from build123d import *
from build123d.topology import SkipClean

# Parameters (mm, degrees)
EXTRUDE_1_DEPTH          = 20
EXTRUDE_2_DEPTH          = 35
FILLET_1_R               = 2
FILLET_2_R               = 2
SKETCH_3_W               = 55
SKETCH_3_H               = 8
EXTRUDE_3_DEPTH          = 20
CUT_EXTRUDE_1_DEPTH      = 81.785122448
FILLET_3_R               = 2
CUT_EXTRUDE_2_DEPTH      = 92.549767886
CUT_EXTRUDE_2_DEPTH_BACK = 92.549767886
SKETCH_6_R               = 3.05
CUT_EXTRUDE_3_DEPTH      = 5.1
FILLET_3_OF_MIRROR_1_R   = 2
CUT_EXTRUDE_4_DEPTH      = 75.837223358
CUT_EXTRUDE_4_DEPTH_BACK = 75.837223358
SKETCH_9_R               = 1.6
SKETCH_10_R              = 3
CUT_EXTRUDE_5_DEPTH      = 3
CUT_EXTRUDE_START        = -2
SKETCH_11_R              = 3
CUT_EXTRUDE_6_DEPTH      = 2
CUT_EXTRUDE_7_DEPTH      = 75.837223358
CUT_EXTRUDE_7_DEPTH_BACK = 75.837223358
SKETCH_12_W              = 29.59816484
SKETCH_12_H              = 37.248372047
SKETCH_12_W_2            = 30.6542071
SKETCH_12_H_2            = 41.472541085
SKETCH_13_W              = 45
SKETCH_13_H              = 8
EXTRUDE_4_DEPTH          = 20
CUT_EXTRUDE_8_DEPTH      = 69.398976601
CUT_EXTRUDE_8_DEPTH_BACK = 69.398976601
SKETCH_14_R              = 2.1
FILLET_5_R               = 1
FILLET_6_R               = 2


with BuildPart() as part:
    # 草图1 → 凸台-拉伸1 (new body)
    with BuildSketch(Plane.XY):
        with BuildLine():
            Line((-24.5, -24.4), (24.5, -24.4))
            Line((24.5, -24.4), (24.5, 15.6))
            ThreePointArc((24.5, 15.6), (0, 23.936691271), (-24.5, 15.6))
            Line((-24.5, 15.6), (-24.5, -24.4))
        make_face()
        with BuildLine():
            Line((-6.480740698, 9.5), (6.480740698, 9.5))
            ThreePointArc((6.480740698, 9.5), (8.131727984, 8.131727984), (9.5, 6.480740698))
            Line((9.5, 6.480740698), (9.5, -6.480740698))
            ThreePointArc((9.5, -6.480740698), (8.131727984, -8.131727984), (6.480740698, -9.5))
            Line((6.480740698, -9.5), (-6.480740698, -9.5))
            ThreePointArc((-6.480740698, -9.5), (-8.131727984, -8.131727984), (-9.5, -6.480740698))
            Line((-9.5, -6.480740698), (-9.5, 6.480740698))
            ThreePointArc((-9.5, 6.480740698), (-8.131727984, 8.131727984), (-6.480740698, 9.5))
        make_face(mode=Mode.SUBTRACT)
    extrude(amount=EXTRUDE_1_DEPTH)

    # 草图2 → 凸台-拉伸2 (add)
    with SkipClean():  # the faces are left unmerged after this step: merging them gives an invalid solid
        with BuildSketch(Plane.XY.offset(20)):
            with BuildLine():
                Line((-20.5, 18.311818868), (-20.5, -20.4))
                Line((-20.5, -20.4), (20.5, -20.4))
                Line((20.5, -20.4), (20.5, 18.311818868))
                ThreePointArc((20.5, 18.311818868), (22.540818317, 17.016117462), (24.5, 15.6))
                Line((24.5, 15.6), (24.5, -24.4))
                Line((24.5, -24.4), (-24.5, -24.4))
                Line((-24.5, -24.4), (-24.5, 15.6))
                ThreePointArc((-24.5, 15.6), (-22.540818317, 17.016117462), (-20.5, 18.311818868))
            make_face()
        extrude(amount=EXTRUDE_2_DEPTH)

    # 圆角1
    fillet_1_edges = [part.edges().sort_by_distance(p)[0] for p in [
        (-24.5, 15.6, 37.5),
        (24.5, 15.6, 37.5),
        (24.5, -24.4, 37.5),
        (-24.5, -24.4, 37.5),
    ]]
    fillet(fillet_1_edges, radius=FILLET_1_R)

    # 圆角2
    fillet_2_edges = [part.edges().sort_by_distance(p)[0] for p in [
        (8.131727984, 8.131727984, 20),
        (0, 9.5, 20),
        (-8.131727984, 8.131727984, 20),
        (-9.5, 0, 20),
        (-8.131727984, -8.131727984, 20),
        (0, -9.5, 20),
        (8.131727984, -8.131727984, 20),
        (9.5, 0, 20),
    ]]
    fillet(fillet_2_edges, radius=FILLET_2_R)

    # 草图3 → 凸台-拉伸3 (add)
    with SkipClean():  # the faces are left unmerged after this step: merging them gives an invalid solid
        with BuildSketch(Plane.ZY.offset(24.5)):
            with Locations((27.5, 10.599820628)):
                Rectangle(SKETCH_3_W, SKETCH_3_H)
            with Locations((27.5, -18.000179372)):
                Rectangle(SKETCH_3_W, SKETCH_3_H)
        extrude_3 = extrude(amount=EXTRUDE_3_DEPTH)

    # 草图4 → 切除-拉伸1 (cut, symmetric)
    with SkipClean():  # the faces are left unmerged after this step: merging them gives an invalid solid
        with BuildSketch(Plane(origin=(0, 14.599820628, 0), x_dir=(1, 0, 0), z_dir=(0, 1, 0))):
            with BuildLine():
                Line((-39.25, -11.75), (-29.75, -11.75))
                ThreePointArc((-29.75, -11.75), (-29.042893219, -12.042893219), (-28.75, -12.75))
                Line((-28.75, -12.75), (-28.75, -17.25))
                ThreePointArc((-28.75, -17.25), (-29.042893219, -17.957106781), (-29.75, -18.25))
                Line((-29.75, -18.25), (-39.25, -18.25))
                ThreePointArc((-39.25, -18.25), (-39.957106781, -17.957106781), (-40.25, -17.25))
                Line((-40.25, -17.25), (-40.25, -12.75))
                ThreePointArc((-40.25, -12.75), (-39.957106781, -12.042893219), (-39.25, -11.75))
            make_face()
            with BuildLine():
                Line((-39.25, -36.75), (-29.75, -36.75))
                ThreePointArc((-29.75, -36.75), (-29.042893219, -37.042893219), (-28.75, -37.75))
                Line((-28.75, -37.75), (-28.75, -42.25))
                ThreePointArc((-28.75, -42.25), (-29.042893219, -42.957106781), (-29.75, -43.25))
                Line((-29.75, -43.25), (-39.25, -43.25))
                ThreePointArc((-39.25, -43.25), (-39.957106781, -42.957106781), (-40.25, -42.25))
                Line((-40.25, -42.25), (-40.25, -37.75))
                ThreePointArc((-40.25, -37.75), (-39.957106781, -37.042893219), (-39.25, -36.75))
            make_face()
        cut_extrude_1 = extrude(amount=CUT_EXTRUDE_1_DEPTH, both=True, mode=Mode.SUBTRACT)

    # 圆角3
    fillet_3_edges = [part.edges().sort_by_distance(p)[0] for p in [
        (-44.5, 6.599820628, 27.5),
        (-44.5, 14.599820628, 27.5),
        (-44.5, -14.000179372, 27.5),
        (-44.5, -22.000179372, 27.5),
    ]]
    fillet(fillet_3_edges, radius=FILLET_3_R)

    # 草图6 → 切除-拉伸2 (cut, two sides: drawn at the far end of the back side and taken through both)
    with BuildSketch(Plane(origin=(24.5, 0, 0), x_dir=(0, 0, -1), z_dir=(1, 0, 0)).offset(-CUT_EXTRUDE_2_DEPTH_BACK)):
        with Locations(Location((-10.4, 0, 0), (0, 0, 270))):
            Circle(SKETCH_6_R)
    extrude(amount=CUT_EXTRUDE_2_DEPTH + CUT_EXTRUDE_2_DEPTH_BACK, mode=Mode.SUBTRACT)

    # 草图7 → 切除-拉伸3 (cut)
    with BuildSketch(Plane(origin=(24.5, 0, 0), x_dir=(0, 0, -1), z_dir=(1, 0, 0))):
        Polygon((-5.4, -2.886751346), (-5.4, 2.886751346), (-10.4, 5.773502692), (-15.4, 2.886751346), (-15.4, -2.886751346), (-10.4, -5.773502692), align=None)
    cut_extrude_3 = extrude(amount=-CUT_EXTRUDE_3_DEPTH, mode=Mode.SUBTRACT)

    # 镜向1: 凸台-拉伸3, 切除-拉伸1, 切除-拉伸3 across plane
    add(extrude_3.mirror(Plane(origin=(0, 0, 0), x_dir=(0, 0, 1), z_dir=(1, 0, 0))))
    add(cut_extrude_1.mirror(Plane(origin=(0, 0, 0), x_dir=(0, 0, 1), z_dir=(1, 0, 0))), mode=Mode.SUBTRACT)
    add(cut_extrude_3.mirror(Plane(origin=(0, 0, 0), x_dir=(0, 0, 1), z_dir=(1, 0, 0))), mode=Mode.SUBTRACT)

    # 圆角3 of 镜向1
    fillet_3_of_mirror_1_edges = [part.edges().sort_by_distance(p)[0] for p in [
        (44.5, 6.599820628, 27.5),
        (44.5, 14.599820628, 27.5),
        (44.5, -14.000179372, 27.5),
        (44.5, -22.000179372, 27.5),
    ]]
    fillet(fillet_3_of_mirror_1_edges, radius=FILLET_3_OF_MIRROR_1_R)

    # 草图9 → 切除-拉伸4 (cut, two sides: drawn at the far end of the back side and taken through both)
    with BuildSketch(Plane(origin=(0, 0, 0), x_dir=(-1, 0, 0), z_dir=(0, 0, -1)).offset(-CUT_EXTRUDE_4_DEPTH_BACK)):
        with Locations((34.5, -18.000179372)):
            Circle(SKETCH_9_R)
        with Locations((34.5, 10.599820628)):
            Circle(SKETCH_9_R)
        with Locations((-34.5, 10.599820628)):
            Circle(SKETCH_9_R)
        with Locations((-34.5, -18.000179372)):
            Circle(SKETCH_9_R)
    extrude(amount=CUT_EXTRUDE_4_DEPTH + CUT_EXTRUDE_4_DEPTH_BACK, mode=Mode.SUBTRACT)

    # 草图10 → 切除-拉伸5 (cut)
    with BuildSketch(Plane(origin=(0, 0, 0), x_dir=(-1, 0, 0), z_dir=(0, 0, -1))):
        with Locations((34.5, 10.599820628)):
            Circle(SKETCH_10_R)
        with Locations((34.5, -18.000179372)):
            Circle(SKETCH_10_R)
        with Locations((-34.5, -18.000179372)):
            Circle(SKETCH_10_R)
        with Locations((-34.5, 10.599820628)):
            Circle(SKETCH_10_R)
    extrude(amount=-CUT_EXTRUDE_5_DEPTH, mode=Mode.SUBTRACT)

    # 草图11 → 切除-拉伸6 (cut)
    with BuildSketch(Plane.XY.offset(55).offset(CUT_EXTRUDE_START)):
        with Locations(Location((34.5, 10.599820628, 0), (0, 0, 180))):
            Circle(SKETCH_11_R)
        with Locations(Location((34.5, -18.000179372, 0), (0, 0, 180))):
            Circle(SKETCH_11_R)
        with Locations(Location((-34.5, -18.000179372, 0), (0, 0, 180))):
            Circle(SKETCH_11_R)
        with Locations(Location((-34.5, 10.599820628, 0), (0, 0, 180))):
            Circle(SKETCH_11_R)
    extrude(amount=CUT_EXTRUDE_6_DEPTH, mode=Mode.SUBTRACT)

    # 草图12 → 切除-拉伸7 (cut, two sides: drawn at the far end of the back side and taken through both)
    with BuildSketch(Plane(origin=(0, 0, 0), x_dir=(-1, 0, 0), z_dir=(0, 0, -1)).offset(-CUT_EXTRUDE_7_DEPTH_BACK)):
        with Locations((-39.29908242, -4.024365395)):
            Rectangle(SKETCH_12_W, SKETCH_12_H)
        with Locations((39.82710355, -6.136449915)):
            Rectangle(SKETCH_12_W_2, SKETCH_12_H_2)
    extrude(amount=CUT_EXTRUDE_7_DEPTH + CUT_EXTRUDE_7_DEPTH_BACK, mode=Mode.SUBTRACT)

    # 草图13 → 凸台-拉伸4 (add)
    with BuildSketch(Plane.XZ.offset(24.4)):
        with Locations((0, 41.9)):
            Rectangle(SKETCH_13_W, SKETCH_13_H)
        with Locations((0, 13.1)):
            Rectangle(SKETCH_13_W, SKETCH_13_H)
    extrude(amount=EXTRUDE_4_DEPTH)

    # 草图14 → 切除-拉伸8 (cut, two sides: drawn at the far end of the back side and taken through both)
    with BuildSketch(Plane.XY.offset(45.9).offset(-CUT_EXTRUDE_8_DEPTH_BACK)):
        with Locations((-10, -34.4)):
            Circle(SKETCH_14_R)
        with Locations((10, -34.4)):
            Circle(SKETCH_14_R)
    extrude(amount=CUT_EXTRUDE_8_DEPTH + CUT_EXTRUDE_8_DEPTH_BACK, mode=Mode.SUBTRACT)

    # 圆角5
    fillet_5_edges = [part.edges().sort_by_distance(p)[0] for p in [
        (0, -44.4, 37.9),
        (0, -44.4, 45.9),
        (0, -44.4, 9.1),
        (0, -44.4, 17.1),
    ]]
    fillet(fillet_5_edges, radius=FILLET_5_R)

    # 圆角6
    # the kernel refuses this fillet: 2 mm, written as the material it adds along each edge
    with BuildSketch(Plane(origin=(-22.5, -24.4, 45.9), x_dir=(0, -1, 0), z_dir=(1, 0, 0))) as fillet_6_piece_1:
        with BuildLine():
            CenterArc((FILLET_6_R, -FILLET_6_R), FILLET_6_R, 90, 90)
            Line((0, -FILLET_6_R), (0, 0))
            Line((0, 0), (FILLET_6_R, 0))
        make_face()
    extrude(amount=45)
    with BuildSketch(Plane(origin=(22.5, -24.4, 9.1), x_dir=(0, 0, -1), z_dir=(-1, 0, 0))) as fillet_6_piece_2:
        with BuildLine():
            CenterArc((FILLET_6_R, FILLET_6_R), FILLET_6_R, 180, 90)
            Line((0, FILLET_6_R), (0, 0))
            Line((0, 0), (FILLET_6_R, 0))
        make_face()
    extrude(amount=45)


solid = part.part
Here's how the part is built. I have some questions about the finished solid (model axes, mm). A direction names the side the tool comes from. Round coordinates to 2 decimals unless told otherwise and drop trailing zeros. Loops run counter-clockwise (first coordinate to the right, second up) from the corner with the lowest first, then second, coordinate; pieces in that order, holes last. Notation, with made-up numbers: (3.5, -6.75) - (14.5, -6.75) arc R23 ccw to (14.5, 29.25) - close; hole circle Ø3 at (-13, 59). An arc over 180 degrees is marked (long way). One line per question, with ' | ' between items. Start each with the question number.
Q1. I want a section at A-A (y = -34.4). Write out the boundary of the cut face in (x, z).
Q2. I want a section at C-C (y = 0). State how many separate pieces and enclosed holes the cut face has, then the cut area to 3 significant figures.
Q3. Will these pins go through, and if not, where does the flat tip stop? pin 1 (3 mm diameter, centred on x = -9.5, z = 30.5, fed in from +Y); pin 2 (2 mm diameter, centred on x = -1.5, z = 51, fed in from -Y); pin 3 (8 mm diameter, centred on y = -32.5, z = 11, fed in from +X); pin 4 (3 mm diameter, centred on y = -33.5, z = 48.5, fed in from -X).
Q4. For faces 1 (the flat face through (0, -24.4, 51)), 2 (the flat face through (21.986, -4.35, 7.935)), 3 (the flat face through (-21.986, -4.31, 12.935)), which set-ups out of +Z, -Z, +X, -X, +Y, -Y let a thin tool reach every point of the face, with its end or its side?
Q5. Please list where these lines run through material, in increasing order: line 1 (Z direction, x = 13.25, y = 0); line 2 (Z direction, x = 8, y = -29); line 3 (X direction, y = -14, z = 31.5). Write a range as [from, to].
Q6. We'd pull the mould along X, two halves only. Please class faces 4 (the cylindrical face through (8.153, -8.11, 8.874)), 5 (the flat face through (22.5, -35, 42)), 6 (the flat face through (22, 0, 15.4)): +X half, -X half, draft (parallel to the pull), parting line (faces both ways), or undercut.
Q7. I want a section at B-B (z = 41). Write out the boundary of the cut face in (x, y).
Q8. I want a section at D-D (z = 21.5). Write out the boundary of the cut face in (x, y).
Response values:
1) outline: (-22.5, 9.1) - (-12.1, 9.1) - (-12.1, 17.1) - (-22.5, 17.1) - close; (-22.5, 37.9) - (-12.1, 37.9) - (-12.1, 45.9) - (-22.5, 45.9) - close; (-7.9, 9.1) - (7.9, 9.1) - (7.9, 17.1) - (-7.9, 17.1) - close; (-7.9, 37.9) - (7.9, 37.9) - (7.9, 45.9) - (-7.9, 45.9) - close; (12.1, 9.1) - (22.5, 9.1) - (22.5, 17.1) - (12.1, 17.1) - close; (12.1, 37.9) - (22.5, 37.9) - (22.5, 45.9) - (12.1, 45.9) - close
2) separate pieces: 4 | enclosed holes: 0 | area: 656 mm²
3) pin 1: stops at y = -20.4 | pin 2: stops at y = -24.4 | pin 3: stops at x = 22.5 | pin 4: passes through
4) face 1: +Z, +X, -X, -Y | face 2: +X | face 3: -X
5) line 1: z = [0, 7.35], [13.45, 20] | line 2: z = [9.1, 17.1], [37.9, 45.9] | line 3: x = [-24.5, -20.5], [20.5, 24.5]
6) face 4: undercut | face 5: +X half | face 6: draft
7) outline: (-24.5, -22.4) arc R2 ccw to (-22.5, -24.4) - (-22.5, -44.4) - (22.5, -44.4) - (22.5, -24.4) arc R2 ccw to (24.5, -22.4) - (24.5, 14.6) arc R2 ccw to (23.68, 16.22) arc R40.17 ccw to (20.5, 18.31) - (20.5, -20.4) - (-20.5, -20.4) - (-20.5, 18.31) arc R40.17 ccw to (-23.68, 16.22) arc R2 ccw to (-24.5, 14.6) - close; hole circle Ø4.2 at (-10, -34.4); hole circle Ø4.2 at (10, -34.4)
8) outline: (-24.5, -22.4) arc R2 ccw to (-22.5, -24.4) - (22.5, -24.4) arc R2 ccw to (24.5, -22.4) - (24.5, 14.6) arc R2 ccw to (23.68, 16.22) arc R40.17 ccw to (20.5, 18.31) - (20.5, -20.4) - (-20.5, -20.4) - (-20.5, 18.31) arc R40.17 ccw to (-23.68, 16.22) arc R2 ccw to (-24.5, 14.6) - close
